Read the model definition and answer for the solid it produces. Units are mm, in the model's axes. A direction names the side the tool comes from. Coordinates: 2 decimals unless noted, no trailing zeros. Loops run counter-clockwise (first coordinate to the right, second up) from the corner with the lowest first, then second, coordinate; pieces in that order, holes last. Notation, with made-up numbers: (57, -21) -> (73, -21) arc R14 cw to (73, -17) -> close; hole circle Ø4 at (-15, -34). An arc over 180 degrees is marked (long way). Answer as a JSON object with one key per item and string values. Group by question number.
1) Section A-A, the plane y = 10.25 is taken. Give the vertices of the cut face in (x, z), plus the area to 3 significant figures.
2) Section D-D, the plane z = -15.5 is taken. Give the vertices of the cut face in (x, y) (1 decimal).
3) Determine the mould class of faces 1 (the face through (-14.8, 1.75, -17.57)), 2 (the face through (-15.875, 1, -12)), 3 (the face through (2.115, 7, -20)) for opening direction X: released by +X, released by -X, zero draft, split by the parting line, or undercut.
4) Flat-ended cylindrical pins translate along their axes: P1, Ø1.2, axis at y = 3.5, z = -9, coming from the +X side; P2, Ø1.5, axis at x = 3.5, z = -14.5, coming from the -Y side; P3, Ø5, axis at x = -7, z = -11.5, coming from the +Y side. Find the tip coordinate at first contact, or state that the pin passes through.
5) Consider probe 1 along Y at (x, z) = (6, -1.75); probe 2 along Z at (x, y) = (-1, 3); probe 3 along Z at (x, y) = (6.5, 15.75). Determine where each line is inside the solid, lowest interval first. Write a range as [from, to].
6) Which of the six approach directions +Z, -Z, +X, -X, +Y, -Y give full straight-line access (tool end or side, diameter ignored) to faces 4 (the face through (13.703, 1, -16)), 5 (the face through (-6, 10, -11.112)), 6 (the face through (-10.497, 8, -12))?
7) Section B-B, the plane z = -4.25 is taken. Give the vertices of the cut face in (x, y).
8) Section C-C, the plane x = -7 is taken. Give the vertices of the cut face in (y, z).
from build123d import *

# Parameters (mm, degrees)
BOSS_EXTRUDE1_DEPTH = 2.0955
SKETCH2_W           = 20.9931
SKETCH2_H           = 1.5875
BOSS_EXTRUDE2_DEPTH = 15.875
BOSS_EXTRUDE3_DEPTH = 1.27
SKETCH5_W           = 0.8636
SKETCH5_H           = 2.1971
BOSS_EXTRUDE4_DEPTH = 15.875
SKETCH6_R           = 1.0795
BOSS_EXTRUDE5_DEPTH = 2.032
BOSS_EXTRUDE6_DEPTH = 2.1717
SKETCH8_W           = 4.2291
SKETCH8_H           = 8.382
BOSS_EXTRUDE7_DEPTH = 2.0955
BOSS_EXTRUDE8_DEPTH = 2.11455


with BuildPart() as part:
    # Sketch1 → Boss-Extrude1 (new body)
    with BuildSketch(Plane(origin=(0, 0, 0), x_dir=(1, 0, 0), z_dir=(0, 1, 0))):
        Polygon((10.541, 0), (15.875, 5.334), (15.875, 12.7), (-15.875, 12.7), (-15.875, 5.334), (-10.541, 0), align=None)
        with BuildLine():
            Line((-6.2103, 7.3787), (-4.7117, 7.3787))
            ThreePointArc((-4.7117, 7.3787), (-2.667, 5.334), (-4.7117, 3.2893))
            Line((-4.7117, 3.2893), (-6.2103, 3.2893))
            ThreePointArc((-6.2103, 3.2893), (-8.255, 5.334), (-6.2103, 7.3787))
        make_face(mode=Mode.SUBTRACT)
        with BuildLine():
            Line((6.2103, 7.3787), (4.7117, 7.3787))
            ThreePointArc((4.7117, 7.3787), (2.667, 5.334), (4.7117, 3.2893))
            Line((4.7117, 3.2893), (6.2103, 3.2893))
            ThreePointArc((6.2103, 3.2893), (8.255, 5.334), (6.2103, 7.3787))
        make_face(mode=Mode.SUBTRACT)
    extrude(amount=BOSS_EXTRUDE1_DEPTH)

    # Sketch2 → Boss-Extrude2 (add)
    with BuildSketch(Plane(origin=(0, 2.0955, 0), x_dir=(1, 0, 0), z_dir=(0, 1, 0))):
        with Locations((0, 11.90625)):
            Rectangle(SKETCH2_W, SKETCH2_H)
    extrude(amount=BOSS_EXTRUDE2_DEPTH)

    # Sketch4 → Boss-Extrude3 (add)
    with BuildSketch(Plane.ZY.offset(10.49655)):
        Polygon((-11.1125, 6.0071), (-7.2009, 2.0955), (-11.1125, 2.0955), align=None)
    boss_extrude3 = extrude(amount=-BOSS_EXTRUDE3_DEPTH)

    # Sketch5 → Boss-Extrude4 (add)
    with BuildSketch(Plane(origin=(0, 17.9705, 0), x_dir=(1, 0, 0), z_dir=(0, 1, 0))):
        with Locations((-1.51765, 10.01395)):
            Rectangle(SKETCH5_W, SKETCH5_H)
    boss_extrude4 = extrude(amount=-BOSS_EXTRUDE4_DEPTH)

    # Sketch6 → Boss-Extrude5 (add)
    with BuildSketch(Plane(origin=(0, 0, -12.7), x_dir=(-1, 0, 0), z_dir=(0, 0, -1))):
        with Locations(Location((4.60375, 14.6431, 0), (0, 0, 180))):
            Circle(SKETCH6_R)
    boss_extrude5 = extrude(amount=BOSS_EXTRUDE5_DEPTH)

    # Sketch7 → Boss-Extrude6 (add)
    with BuildSketch(Plane.ZY.offset(15.875)):
        Polygon((-12.7, 0), (-19.05, 0), (-19.05, 2.0955), (-16.0401, 1.397), (-12.7, 2.0955), align=None)
    boss_extrude6 = extrude(amount=-BOSS_EXTRUDE6_DEPTH)

    # Mirror1: Boss-Extrude3, Boss-Extrude4, Boss-Extrude5, Boss-Extrude6 across plane
    add(boss_extrude3.mirror(Plane(origin=(0, 0, 0), x_dir=(0, 0, 1), z_dir=(1, 0, 0))))
    add(boss_extrude4.mirror(Plane(origin=(0, 0, 0), x_dir=(0, 0, 1), z_dir=(1, 0, 0))))
    add(boss_extrude5.mirror(Plane(origin=(0, 0, 0), x_dir=(0, 0, 1), z_dir=(1, 0, 0))))
    add(boss_extrude6.mirror(Plane(origin=(0, 0, 0), x_dir=(0, 0, 1), z_dir=(1, 0, 0))))

    # Sketch8 → Boss-Extrude7 (add)
    with BuildSketch(Plane(origin=(0, 0, 0), x_dir=(-1, 0, 0), z_dir=(0, -1, 0))):
        with Locations((0, 16.891)):
            Rectangle(SKETCH8_W, SKETCH8_H)
    extrude(amount=-BOSS_EXTRUDE7_DEPTH)

    # Sketch9 → Boss-Extrude8 (add, symmetric)
    with BuildSketch(Plane(origin=(0, 0, 0), x_dir=(0, 0, -1), z_dir=(1, 0, 0))):
        Polygon((21.082, 2.0955), (21.123652242, 21.7297), (20.158454414, 21.731747583), (19.304, 20.057156461), (19.265895913, 2.0955), align=None)
    extrude(amount=BOSS_EXTRUDE8_DEPTH, both=True)


solid = part.part
Determined:
{
 "1": {"outline": "(-10.5, -12.7) -> (10.5, -12.7) -> (10.5, -11.11) -> (1.95, -11.11) -> (1.95, -8.92) -> (1.09, -8.92) -> (1.09, -11.11) -> (-1.09, -11.11) -> (-1.09, -8.92) -> (-1.95, -8.92) -> (-1.95, -11.11) -> (-10.5, -11.11) -> close; (-2.11, -21.1) -> (2.11, -21.1) -> (2.11, -19.28) -> (-2.11, -19.28) -> close", "area": "44.8 mm²"},
 "2": {"outline": "(-15.9, 0) -> (-13.7, 0) -> (-13.7, 1.5) -> (-15.9, 1.5) -> close; (-2.1, 0) -> (2.1, 0) -> (2.1, 2.1) -> (-2.1, 2.1) -> close; (13.7, 0) -> (15.9, 0) -> (15.9, 1.5) -> (13.7, 1.5) -> close"},
 "3": {"face 1": "zero draft", "face 2": "released by -X", "face 3": "undercut"},
 "4": {"P1": "x = 10.5", "P2": "y = 13.62", "P3": "y = 17.97"},
 "5": {"probe 1": "[0, 2.1]", "probe 2": "[-21.08, -19.27], [-12.7, -11.11]", "probe 3": "[-12.7, -11.11]"},
 "6": {"face 4": "-Z, +Y, -Y", "face 5": "+Z, +Y", "face 6": "+Z, -Z, -X, +Y"},
 "7": {"outline": "(-14.79, 0) -> (-7.94, 0) -> (-7.94, 2.1) -> (-14.79, 2.1) -> close; (-2.98, 0) -> (2.98, 0) -> (2.98, 2.1) -> (-2.98, 2.1) -> close; (7.94, 0) -> (14.79, 0) -> (14.79, 2.1) -> (7.94, 2.1) -> close"},
 "8": {"outline": "(0, -12.7) -> (17.97, -12.7) -> (17.97, -11.11) -> (2.1, -11.11) -> (2.1, -7.22) -> (0, -7.22) -> close; (0, -3.45) -> (2.1, -3.45) -> (2.1, 0) -> (0, 0) -> close"}
}
